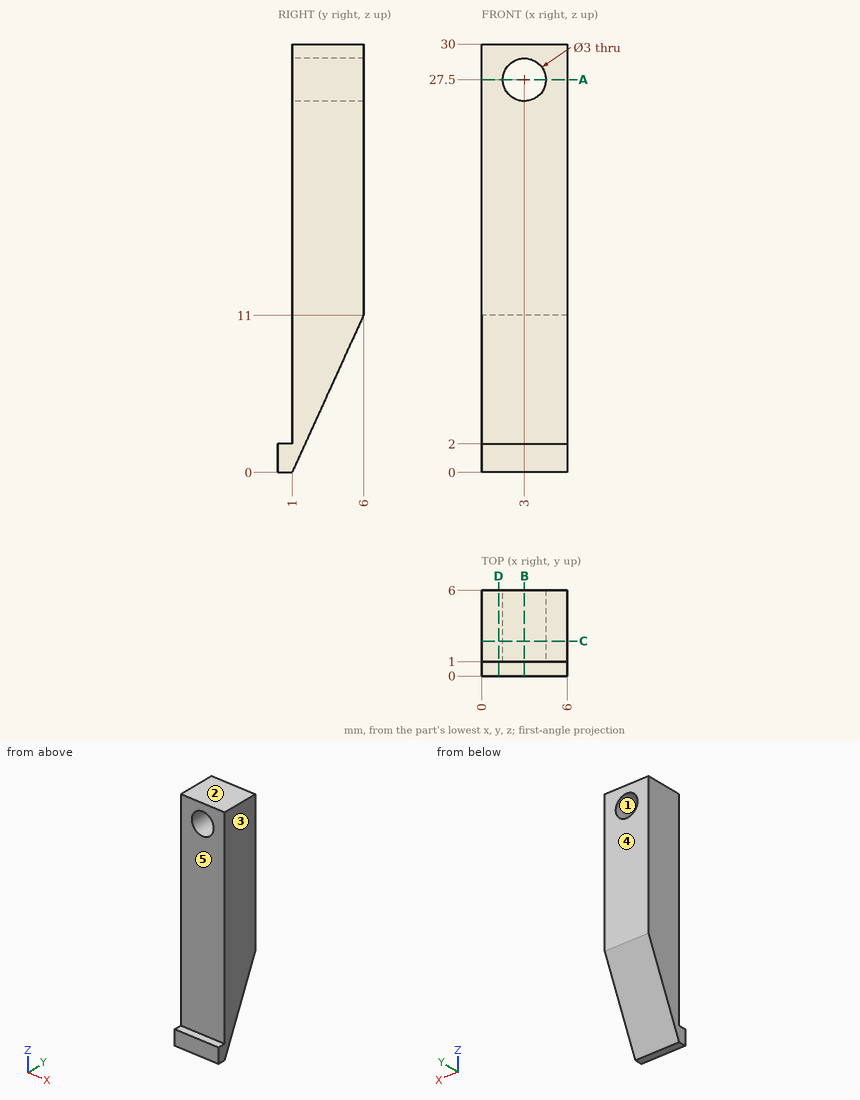
The figure shows three views and two pictorial views of one solid part (mm, origin at its lowest corner). Answer the questions. A direction names the side the tool comes from. Give positions to 0.01 mm unless a question says otherwise; leave off trailing zeros. Write each loop counter-clockwise with the first axis right and the second up, starting at its lowest first coordinate (ties: lowest second). Pieces come first, ordered by that corner, then holes. Notation, with made-up numbers: M -35.75,15.25 L -22.75,15.25 A18 cw -22.75,22.25 Z; hole C 88,72.25 d11. An arc over 180 degrees is marked long. One line per item, written item: value. Start each with the question number.
(1) Find the intervals of material crossed by line 1 (Y direction, x = 3.7, z = 14.5); line 2 (Z direction, x = 4.1, y = 4.5) (1 decimal); line 3 (Z direction, x = 3, y = 4.15) (1 decimal), in increasing order.
(2) Find section D-D (x = 1.2). Determine the outline of the cut face in (y, z).
(3) Flat-ended cylindrical pins translate along their axes: pin 1 Ø1 at (x, z) = (4, 26.5) entering from +Y; pin 2 Ø2 at (x, z) = (4, 4) entering from -Y. Find the tip coordinate at first contact, or state that the pin passes through.
(4) Find section B-B (x = 3). Determine the outline of the cut face in (y, z).
(5) Find section A-A (z = 27.5). Determine the outline of the cut face in (x, y).
(6) Find section C-C (y = 2.45). Determine the outline of the cut face in (x, z), plus the area to 3 significant figures.
(7) A tool of negligible diameter and unlimited length cuts with its end or side. For the marked faces 4 and 5, from which of +Z, -Z, +X, -X, +Y, -Y can it reach the whole face along a straight path? Write none if from no direction.
(8) Determine the mould class of the marked faces 1, 2 and 3 for opening direction X: pulls with the +X half, pulls with the -X half, needs draft (parallel to the pull), parting line crosses it, or undercut.
Results below:
1. line 1: y = 1 to 6
1. line 2: z = 7.7 to 26.5, 28.5 to 30
1. line 3: z = 6.9 to 26, 29 to 30
2. outline: M 0,0 L 1,0 L 6,11 L 6,30 L 1,30 L 1,2 L 0,2 Z
3. pin 1: stops at y = 6
3. pin 2: stops at y = 1
4. outline: M 0,0 L 1,0 L 6,11 L 6,26 L 1,26 L 1,2 L 0,2 Z; M 1,29 L 6,29 L 6,30 L 1,30 Z
5. outline: M 0,1 L 1.5,1 L 1.5,6 L 0,6 Z; M 4.5,1 L 6,1 L 6,6 L 4.5,6 Z
6. outline: M 0,3.19 L 6,3.19 L 6,30 L 0,30 Z; hole C 3,27.5 d3
6. area: 154 mm^2
7. face 4: +Z, -Z, +X, -X, +Y
7. face 5: +Z, +X, -X, -Y
8. face 1: undercut
8. face 2: needs draft
8. face 3: pulls with the +X half
